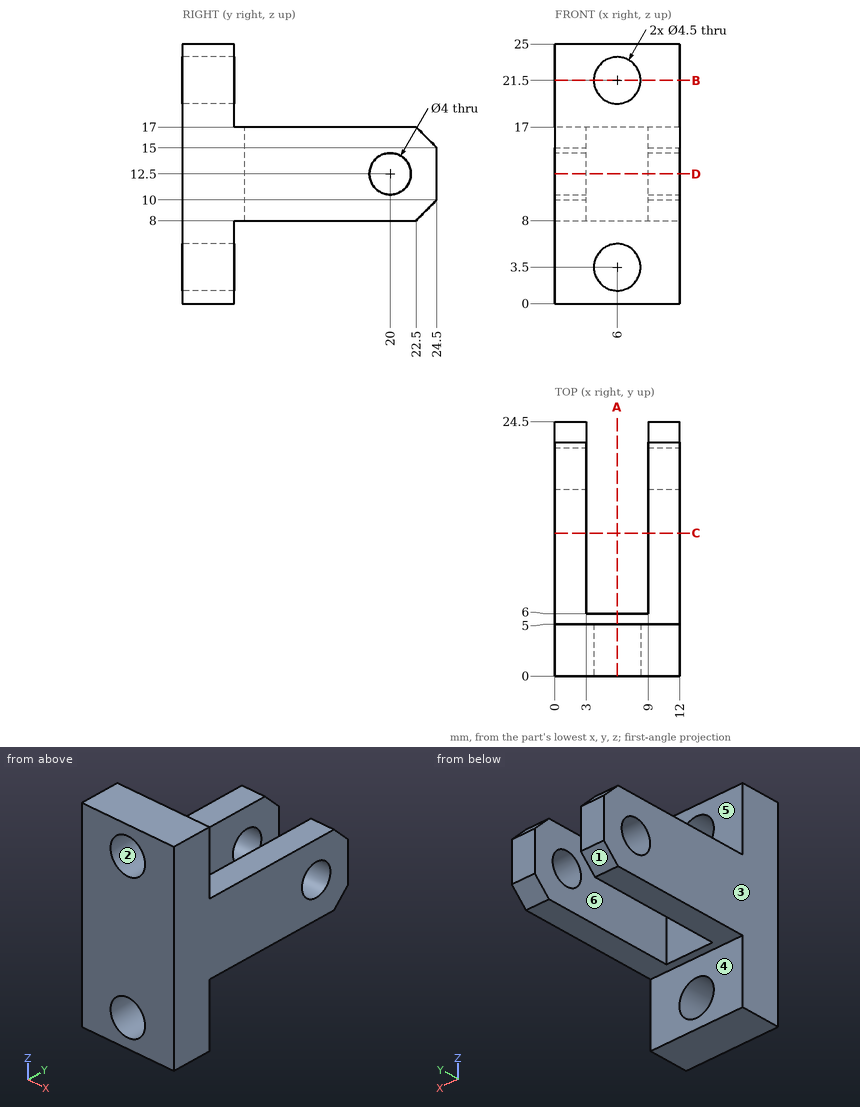
Input: dimensioned drawing with shaded views. Units: mm. Origin: part minimum x, y, z. A direction names the side the tool comes from. Give positions to 0.01 mm unless a question says otherwise; leave off trailing zeros. Loops run counter-clockwise (first coordinate to the right, second up) from the corner with the lowest first, then second, coordinate; pieces in that order, holes last. Notation, with made-up numbers: M 21.25,-25.75 L 79.25,-25.75 A11 ccw 79.25,-10.75 Z; hole C -32.5,-20 d3. An arc over 180 degrees is marked long. Put each result on its own line as item: value.
1) Mould query, pull axis X, two halves, no side actions, for the marked faces 1, 2 and 3. Classes: released by +X, released by -X, zero draft, split by the parting line, or undercut.
Computed values:
face 1: zero draft
face 2: undercut
face 3: released by -X
2) Material intervals for L1, parallel to Z at x = 6, y = 2.5; L2, parallel to Z at x = 10.2, y = 20; L3, parallel to X at y = 9.5, z = 12, sorted ascending. Write a range as from..to.
Computed values:
L1: z = 0..1.25, 5.75..19.25, 23.75..25
L2: z = 8..10.5, 14.5..17
L3: x = 0..3, 9..12
3) Cut plane A-A, the plane x = 6. Return the cut outline in (y, z).
Computed values:
outline: M 0,0 L 5,0 L 5,1.25 L 0,1.25 Z; M 0,5.75 L 5,5.75 L 5,8 L 6,8 L 6,17 L 5,17 L 5,19.25 L 0,19.25 Z; M 0,23.75 L 5,23.75 L 5,25 L 0,25 Z
4) Reachability of the marked faces 4, 5 and 6 from +Z, -Z, +X, -X, +Y, -Y: full face, straight path, thin tool, end or side. Return the list, or none.
Computed values:
face 4: -Z, +X, -X, +Y
face 5: +Z, +X, -X, +Y
face 6: +Z, -Z, +Y
5) Cut plane C-C, the plane y = 13.75. Return the cut outline in (x, z), plus the area to 3 significant figures.
Computed values:
outline: M 0,8 L 3,8 L 3,17 L 0,17 Z; M 9,8 L 12,8 L 12,17 L 9,17 Z
area: 54.0 mm^2
6) Cut plane B-B, the plane z = 21.5. Return the cut outline in (x, y), plus the area to 3 significant figures.
Computed values:
outline: M 0,0 L 3.75,0 L 3.75,5 L 0,5 Z; M 8.25,0 L 12,0 L 12,5 L 8.25,5 Z
area: 37.5 mm^2
7) First-contact query: P1, Ø2.5, axis at x = 6, z = 21.5, coming from the -Y side; P2, Ø3.5, axis at x = 4.5, y = 13, coming from the +Z side; P3, Ø1.5, axis at y = 5, z = 4.5, coming from the -X side; P4, Ø2.5, axis at x = 5.5, z = 19.5, coming from the +Y side. Flat tips, straight axial feed; report the tip coordinate or a pass-through.
Computed values:
P1: passes through
P2: stops at z = 17
P3: stops at x = 0
P4: stops at y = 5
8) Cut plane D-D, the plane z = 12.5. Return the cut outline in (x, y), plus the area to 3 significant figures.
Computed values:
outline: M 0,0 L 12,0 L 12,18 L 9,18 L 9,6 L 3,6 L 3,18 L 0,18 Z; M 0,22 L 3,22 L 3,24.5 L 0,24.5 Z; M 9,22 L 12,22 L 12,24.5 L 9,24.5 Z
area: 159 mm^2
